Read the model definition and answer for the solid it produces. Units are mm, in the model's axes. A direction names the side the tool comes from. Coordinates: 2 decimals unless noted, no trailing zeros. Order: outer loops, then holes, each group sorted by start corner. A loop starts at its lowest first (then second) coordinate and runs counter-clockwise, first axis right, second up. Notation, with made-up numbers: (54, 52.5) -> (88, 52.5) arc R27 ccw to (88, 84.5) -> close; hole circle Ø6 at (31.25, 20.5). An arc over 180 degrees is marked (long way). Return JSON: item names as keys, results as strings. Group by question number.
Autodesk Inventor part; units mm, degrees
ref_plane "YZ Plane" through (0, 0, 0) normal (1, 0, 0) x (0, 1, 0)
ref_plane "XZ Plane" through (0, 0, 0) normal (0, 1, 0) x (-1, 0, 0)
ref_plane "XY Plane" through (0, 0, 0) normal (0, 0, 1) x (1, 0, 0)
sketch "Sketch1" plane through (0, 0, 0) normal (1, 0, 0) x (0, 1, 0)
  line L0 (-30, -15.5) -> (30, -15.5)
  line L1 (30, -15.5) -> (30, 15.5)
  line L2 (30, 15.5) -> (-30, 15.5)
  line L3 (-30, 15.5) -> (-30, -15.5)
  line L4 (-30, -15.5) -> (30, 15.5) construction
  line L5 (30, -15.5) -> (-30, 15.5) construction
  point P0 (0, 0)
  dimension "d0" = 60
  dimension "d1" = 31
extrude "Extrusion1" add sketch "Sketch1" along normal blind 5
fillet "Fillet1" radius 4 4 edges at (2.5, 30, 15.5) (2.5, 30, -15.5) (2.5, -30, -15.5) (2.5, -30, 15.5)
sketch "Sketch2" plane through (5, 0, 0) normal (1, 0, 0) x (0, 0, -1)
  line L0 (-15.5, 26) -> (-15.5, -26)
  line L1 (11.5, 30) -> (-11.5, 30)
  point P0 (0, 0)
  point P1 (-9, 25.0416)
  point P2 (-9, -24.9584)
  point P3 (-2.5, 25.0416)
  point P4 (-2.5, -24.9584)
  point P5 (4, 25.0416)
  point P6 (4, -24.9584)
  point P7 (10.5, 25.0416)
  point P8 (10.5, -24.9584)
  dimension "d5" = 6.5
  dimension "d8" = 50
  dimension "d11" = 6.5
hole "Hole1" at (5, 25.0416, 9) at (5, -24.9584, 9) at (5, 25.0416, 2.5) at (5, -24.9584, 2.5) at (5, 25.0416, -4) at (5, -24.9584, -4) at (5, 25.0416, -10.5) at (5, -24.9584, -10.5) direction (-1, 0, 0) diameter 3.242 depth 11.8 tip angle 118 countersink diameter 4 countersink angle 90
sketch "Sketch3" plane through (5, 0, 0) normal (1, 0, 0) x (0, 0, -1)
  circle A0 centre (0, 0) radius 4
  dimension "d21" = 8
extrude "Extrusion2" cut sketch "Sketch3" against normal blind 5
sketch "Sketch4" plane through (0, -26, 15.5) normal (0, 0, 1) x (1, 0, 0)
  line L0 (0, 0) -> (0, 52)
  line L1 (0, 6) -> (-45, 6)
  line L2 (-45, 6) -> (-45, 46)
  line L3 (-45, 46) -> (0, 46)
  line L4 (0, 46) -> (0, 6)
  line L5 (5, 52) -> (5, 0)
  line L6 (0, 26) -> (-7.0205, 26) construction
  dimension "d24" = 50
  dimension "d25" = 40
extrude "Extrusion3" add sketch "Sketch4" against normal up to surface (31 mm away)
sketch "Sketch5" plane through (-45, -20, 15.5) normal (-1, 0, 0) x (0, 0, 1)
  circle A0 centre (-15.5, 20) radius 5.4211
extrude "Extrusion4" add sketch "Sketch5" along normal blind 6
sketch "Sketch6" plane through (5, 0, 0) normal (1, 0, 0) x (0, 0, -1)
  circle A0 centre (0, 0) radius 11.0071
extrude "Extrusion5" add sketch "Sketch6" along normal blind 61
chamfer "Chamfer1" distance 10.5 angle 45 1 edges at (66, 0, 11.0071)
properties part number "GT9S Extruder"
1. Straight lines are drawn through the part: L1, parallel to Y at x = 2.85, z = -10.5; L2, parallel to Z at x = 3, y = -24.5; L3, parallel to Y at x = 2.3, z = 0. For each, find the intervals that lie inside material, in ascending order.
2. Find section C-C on x = -6. Determine the outline of the cut face in (y, z).
3. Which of the six approach directions +Z, -Z, +X, -X, +Y, -Y give full straight-line access (tool end or side, diameter ignored) to faces 5 (the face through (-20, 0, -15.5)), 6 (the face through (-22, -20, 0)), 7 (the face through (29.896, 10.745, 2.386))?
4. Find section B-B on y = 18. Determine the outline of the cut face in (x, z), and give its area (3 significant figures).
5. For a pull along Z with two mould halves and no side action, classify faces 1 (the face through (63.01, 3.414, 0.758)), 2 (the face through (2.535, -3.905, 0.867)), 3 (the face through (2.535, -28.797, 14.359)), 4 (the face through (-45, -5, 4)) as released by +Z, released by -Z, zero draft, split by the parting line, or undercut.
6. Given pin 1 (15.5 mm diameter, centred on y = 10.5, z = -0.5, fed in from +X); pin 2 (2 mm diameter, centred on y = -9.5, z = 11, fed in from -X); pin 3 (2 mm diameter, centred on x = -2, z = -9.5, fed in from +Y); pin 4 (3 mm diameter, centred on y = 25.04, z = -10.5, fed in from +X), each flat-ended and moving along its own axis, determine where each tip first touches the part or whether it passes through.
7. Find section A-A on z = 2.5. Give the number of separate pieces and of enclosed holes in the cut face, and give its area (3 significant figures).
Result:
{
 "1": {"L1": "-30 to -26.58, -23.34 to 23.42, 26.66 to 30", "L2": "-15.5 to -12.05, -8.95 to -5.55, -2.45 to 0.95, 4.05 to 7.45, 10.55 to 15.5", "L3": "-30 to -4, 4 to 30"},
 "2": {"outline": "(-20, -15.5) -> (20, -15.5) -> (20, 15.5) -> (-20, 15.5) -> close"},
 "3": {"face 5": "-Z, +X, -X, +Y, -Y", "face 6": "+Z, -Z, -X, -Y", "face 7": "+X"},
 "4": {"outline": "(-45, -15.5) -> (5, -15.5) -> (5, 15.5) -> (-45, 15.5) -> close", "area": "1,550 mm^2"},
 "5": {"face 1": "split by the parting line", "face 2": "undercut", "face 3": "released by +Z", "face 4": "zero draft"},
 "6": {"pin 1": "x = 63.75", "pin 2": "x = -45", "pin 3": "y = 20", "pin 4": "through"},
 "7": {"separate pieces": "3", "enclosed holes": "1", "area": "3,280 mm^2"}
}
